Check sheet for the modelled part. Datum: model origin and axes. Units: mm. A direction names the side the tool comes from. Round coordinates to 2 decimals unless told otherwise and drop trailing zeros. Loops run counter-clockwise (first coordinate to the right, second up) from the corner with the lowest first, then second, coordinate; pieces in that order, holes last. Notation, with made-up numbers: (42.5, 68) - (54.5, 68) arc R23 cw to (54.5, 86) - close; hole circle Ø8 at (3.25, 56.5). An arc over 180 degrees is marked (long way). Put each result on its own line as item: value. Start each with the question number.
```python
from build123d import *

# Parameters (mm, degrees)
SKETCH_1_R          = 7.5
EXTRUDE_1_DEPTH     = 3
SKETCH_2_W          = 25
SKETCH_2_H          = 4
EXTRUDE_2_DEPTH     = 10
FILLET_1_R          = 3
SKETCH_8_R          = 8.25
CUT_EXTRUDE_2_DEPTH = 0.8
SCALE_1_SCALE       = 0.6
SKETCH_3_R          = 1.6
CUT_EXTRUDE_3_DEPTH = 5


with BuildPart() as part:
    # 草图1 → 凸台-拉伸1 (new body)
    with BuildSketch(Plane(origin=(0, 0, 0), x_dir=(0, 0, -1), z_dir=(1, 0, 0))):
        with BuildLine():
            Line((-12.5, 0), (-12.5, 35))
            Line((-12.5, 35), (12.5, 35))
            Line((12.5, 35), (12.5, 0))
            ThreePointArc((12.5, 0), (0, -12.5), (-12.5, 0))
        make_face()
        Circle(SKETCH_1_R, mode=Mode.SUBTRACT)
    extrude(amount=EXTRUDE_1_DEPTH)

    # 草图2 → 凸台-拉伸2 (add)
    with BuildSketch(Plane.ZY):
        with Locations((0, 33)):
            Rectangle(SKETCH_2_W, SKETCH_2_H)
    extrude(amount=EXTRUDE_2_DEPTH)

    # 圆角1
    fillet_1_edges = [part.edges().sort_by_distance(p)[0] for p in [
        (-10, 33, 12.5),
        (-10, 33, -12.5),
    ]]
    fillet(fillet_1_edges, radius=FILLET_1_R)

    # 草图8 → 切除-拉伸2 (cut)
    with BuildSketch(Plane(origin=(3, 0, 0), x_dir=(0, 0, -1), z_dir=(1, 0, 0))):
        Circle(SKETCH_8_R)
    extrude(amount=-CUT_EXTRUDE_2_DEPTH, mode=Mode.SUBTRACT)


with BuildPart() as part_1:
    # 缩放比例1: scaled about (-0.181266262, 19.683257287, 0)
    add(part.part.scale(SCALE_1_SCALE).moved(Location((-0.072506505, 7.873302915, 0))))

    # 草图3 → 切除-拉伸3 (cut)
    with BuildSketch(Plane(origin=(0, 28.873302915, 0), x_dir=(1, 0, 0), z_dir=(0, 1, 0))):
        with Locations(Location((-4, 4, 0), (0, 0, 270))):
            Circle(SKETCH_3_R)
        with Locations(Location((-4, -4, 0), (0, 0, 270))):
            Circle(SKETCH_3_R)
    extrude(amount=-CUT_EXTRUDE_3_DEPTH, mode=Mode.SUBTRACT)


solid = part_1.part
```
Q1. Depth check by flat-ended pin: pin 1 Ø6 at (y, z) = (7.87, 0) entering from -X; pin 2 Ø3 at (y, z) = (16, 4) entering from -X; pin 3 Ø3 at (x, z) = (-2.5, 2) entering from -Y. Enter the tip coordinate at first touch or a pass-through.
Q2. Cross-section at A-A on x = -4. Enter the section's corners in (y, z).
Q3. Material ranges on line 1 (Y direction, x = 1, z = 0); line 2 (Z direction, x = -3.5, y = 27.75); line 3 (X direction, y = 27.25, z = -4), recorded low to high. Write a range as from..to.
Q4. Cross-section at C-C on x = 0.75. Enter the section's corners in (y, z).
Q5. Cross-section at B-B on z = 0. Enter the section's corners in (x, y).
Q6. Set-up check for faces 1 (the face through (0.1, 20.6, 7.5)), 2 (the face through (-3, 26.473, 0)): record each of +Z, -Z, +X, -X, +Y, -Y from which the full face is reachable in a straight line by a thin tool's end or side.
Q7. Draft check along Y on faces 3 (the face through (1.49, 3.04, 1.07)), 4 (the face through (-2, 28.873, 0)), 5 (the face through (-0.073, 17, 0)). Enter one of: +Y half, -Y half, draft (parallel to the pull), parting line (faces both ways), or undercut.
Q8. Cross-section at D-D on y = 24. Enter the section's corners in (x, z).
Answer list:
1. pin 1: passes through
1. pin 2: stops at x = -0.07
1. pin 3: stops at y = 26.47
2. outline: (26.47, -7.5) - (28.87, -7.5) - (28.87, -5.6) - (26.47, -5.6) - close; (26.47, -2.4) - (28.87, -2.4) - (28.87, 2.4) - (26.47, 2.4) - close; (26.47, 5.6) - (28.87, 5.6) - (28.87, 7.5) - (26.47, 7.5) - close
3. line 1: y = 0.37..3.37, 12.37..28.87
3. line 2: z = -7.5..-5.52, -2.48..2.48, 5.52..7.5
3. line 3: x = -6.07..-5.6, -2.4..1.73
4. outline: (7.87, -7.5) - (28.87, -7.5) - (28.87, 7.5) - (7.87, 7.5) arc R7.5 ccw to start; hole circle Ø9 at (7.87, 0)
5. outline: (-6.07, 26.47) - (-0.07, 26.47) - (-0.07, 12.37) - (1.25, 12.37) - (1.25, 12.82) - (1.73, 12.82) - (1.73, 28.87) - (-6.07, 28.87) - close; (-0.07, 0.37) - (1.73, 0.37) - (1.73, 2.92) - (1.25, 2.92) - (1.25, 3.37) - (-0.07, 3.37) - close
6. face 1: +Z, +X, -X, +Y, -Y
6. face 2: +Z, -Z, -X, -Y
7. face 3: undercut
7. face 4: +Y half
7. face 5: draft
8. outline: (-0.07, -7.5) - (1.73, -7.5) - (1.73, 7.5) - (-0.07, 7.5) - close
